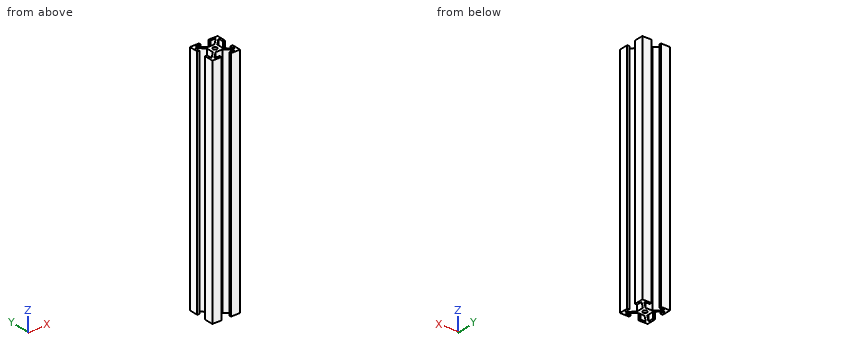
```python
from build123d import *

# Parameters (mm, degrees)
F0_R            = 1.5
F1_DEPTH        = 170
F1_COPIES_COUNT = 4


# Not quite as in the source:
# - a pattern or mirror of a feature is missing from the dataset's text; its kind, count and spacing are read off the source's solid
# - a feature names something its author has since deleted; it is built from what else it names


with BuildPart() as f1:
    # F0 (on Top) → F1 (new body)
    with BuildSketch(Plane.XY):
        Polygon((-3.66, -3.66), (3.66, -3.66), (3.66, 3.66), (-2.5993398282, 3.66), (-3.66, 2.5993398282), align=None)
        Circle(F0_R, mode=Mode.SUBTRACT)
        Polygon((-8.5, 7.4393398282), (-3.66, 2.5993398282), (-2.5993398282, 3.66), (-7.4393398282, 8.5), (-3.5, 8.5), (-3.5, 10), (-10, 10), (-10, 3.5), (-8.5, 3.5), align=None)
    extrude(amount=F1_DEPTH)

    # F1_copies: F1 ×4 about axis
    f1_copies_axis = Axis((0, 0, 0), (0, 0, 1))


with BuildPart() as f1_1:
    add(f1.part)
    for i in range(1, F1_COPIES_COUNT):
        add(f1.part.rotate(f1_copies_axis, i * 360 / F1_COPIES_COUNT))


solid = f1_1.part
```
Geometry check sheet. Reference: the model listing, model coordinates, mm. Give positions to 0.01 mm unless a question says otherwise; leave off trailing zeros. Order: outer loops, then holes, each group sorted by start corner. A loop starts at its lowest first (then second) coordinate and runs counter-clockwise, first axis right, second up.
1. Thickness scan on L1, parallel to Y at x = -6.5, z = 155; L2, parallel to Y at x = 0, z = 74.5; L3, parallel to Y at x = -7.25, z = 159. Record the ranges inside material, lowest first.
2. Gauge pin test, flat ends, axial feed: pin 1 Ø4 at (y, z) = (0, 44) entering from -X; pin 2 Ø2 at (x, z) = (1.5, 59.5) entering from -Y. Record the tip position at first contact, or that the pin passes through.
3. Section check A-A, the plane x = 0. Enter the section's corners in (y, z), and give its area (3 significant figures).
Values follow:
1. L1: y = -10 to -8.5, -7.56 to -5.44, 5.44 to 7.56, 8.5 to 10
1. L2: y = -3.66 to -1.5, 1.5 to 3.66
1. L3: y = -10 to -8.5, -8.31 to -6.19, 6.19 to 8.31, 8.5 to 10
2. pin 1: stops at x = -3.66
2. pin 2: stops at y = -3.66
3. outline: (-3.66, 0) - (-1.5, 0) - (-1.5, 170) - (-3.66, 170) - close; (1.5, 0) - (3.66, 0) - (3.66, 170) - (1.5, 170) - close
3. area: 734 mm2
